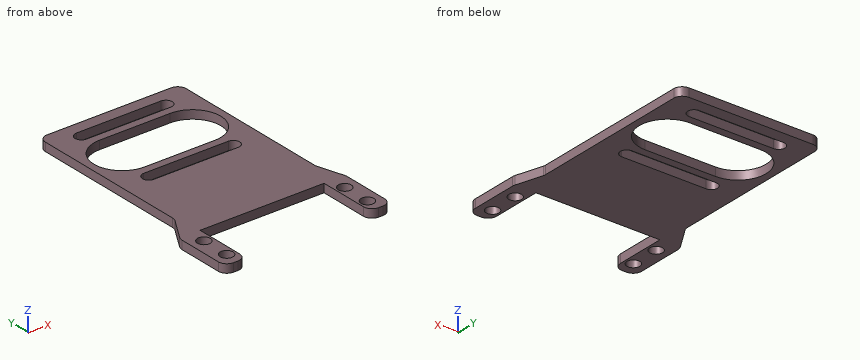
```python
from build123d import *

# Parameters (mm, degrees)
SKETCH1_R           = 2.3
BOSS_EXTRUDE1_DEPTH = 3
FILLET1_R           = 3


with BuildPart() as part:
    # Sketch1 → Boss-Extrude1 (new body)
    with BuildSketch(Plane.XY):
        Polygon((7.5, -20.05), (0, -20.05), (0, 0), (6, 10), (6, 70.5), (56, 70.5), (56, 10), (59, 0), (59, -20.05), (51.5, -20.05), (51.5, 0.5), (7.5, 0.5), align=None)
        with Locations((4.5, -15.05)):
            Circle(SKETCH1_R, mode=Mode.SUBTRACT)
        with Locations((4.5, -4.95)):
            Circle(SKETCH1_R, mode=Mode.SUBTRACT)
        with Locations((54.5, -15.05)):
            Circle(SKETCH1_R, mode=Mode.SUBTRACT)
        with Locations((54.5, -4.95)):
            Circle(SKETCH1_R, mode=Mode.SUBTRACT)
        with BuildLine():
            Line((18.5, 59), (43.5, 59))
            ThreePointArc((43.5, 59), (53.5, 49), (43.5, 39))
            Line((43.5, 39), (18.5, 39))
            ThreePointArc((18.5, 39), (8.5, 49), (18.5, 59))
        make_face(mode=Mode.SUBTRACT)
        with BuildLine():
            Line((16, 66.25), (46, 66.25))
            ThreePointArc((46, 66.25), (48.25, 64), (46, 61.75))
            Line((46, 61.75), (16, 61.75))
            ThreePointArc((16, 61.75), (13.75, 64), (16, 66.25))
        make_face(mode=Mode.SUBTRACT)
        with BuildLine():
            Line((16, 36.25), (46, 36.25))
            ThreePointArc((46, 36.25), (48.25, 34), (46, 31.75))
            Line((46, 31.75), (16, 31.75))
            ThreePointArc((16, 31.75), (13.75, 34), (16, 36.25))
        make_face(mode=Mode.SUBTRACT)
    extrude(amount=BOSS_EXTRUDE1_DEPTH)

    # Fillet1
    fillet1_edges = [part.edges().sort_by_distance(p)[0] for p in [
        (0, 0, 1.5),
        (6, 10, 1.5),
        (6, 70.5, 1.5),
        (56, 70.5, 1.5),
        (56, 10, 1.5),
        (59, 0, 1.5),
        (59, -20.05, 1.5),
        (51.5, -20.05, 1.5),
        (7.5, -20.05, 1.5),
        (0, -20.05, 1.5),
    ]]
    fillet(fillet1_edges, radius=FILLET1_R)


solid = part.part
```
CAD build for the part. Positions are in the model's coordinates, mm. Round coordinates to 2 decimals unless told otherwise and drop trailing zeros. Loops run counter-clockwise (first coordinate to the right, second up) from the corner with the lowest first, then second, coordinate; pieces in that order, holes last. Notation, with made-up numbers: M 58,-28.75 L 82,-28.75 A11 ccw 82,-24.75 Z; hole C 71,-18.75 d2. An arc over 180 degrees is marked long. Use a Markdown table: item, result. Add a question column.
(1) Cut at A-A (y = 64). Give the cut face in (x, z), and give its area (3 significant figures).
(2) Cut at B-B (x = 22.5). Give the cut face in (y, z).
(3) Cut at C-C (y = -4.95). Give the cut face in (x, z), and give its area (3 significant figures).
(4) Flat gauge pins, fed straight in: pin 1 (1.5 mm diameter, centred on x = 34, z = 1, fed in from -Y); pin 2 (3 mm diameter, centred on x = 4.5, y = -15.05, fed in from +Z); pin 3 (1.5 mm diameter, centred on y = 37.5, z = 2, fed in from -X). Where does each tip first touch, or does it go through?
(5) Drill centre lines: line 1 (Y direction, x = 36, z = 2.55); line 2 (Y direction, x = 4.5, z = 0.95); line 3 (X direction, y = -10, z = 1.15). Where is each one in solid material? Low to high.
(6) Cut at D-D (x = 10.5). Give the cut face in (y, z).
Geometry says:
| question | item | result |
|---|---|---|
| 1 | outline | M 6,0 L 13.75,0 L 13.75,3 L 6,3 Z; M 48.25,0 L 56,0 L 56,3 L 48.25,3 Z |
| 1 | area | 46.5 mm² |
| 2 | outline | M 0.5,0 L 31.75,0 L 31.75,3 L 0.5,3 Z; M 36.25,0 L 39,0 L 39,3 L 36.25,3 Z; M 59,0 L 61.75,0 L 61.75,3 L 59,3 Z; M 66.25,0 L 70.5,0 L 70.5,3 L 66.25,3 Z |
| 3 | outline | M 0,0 L 2.2,0 L 2.2,3 L 0,3 Z; M 6.8,0 L 7.5,0 L 7.5,3 L 6.8,3 Z; M 51.5,0 L 52.2,0 L 52.2,3 L 51.5,3 Z; M 56.8,0 L 59,0 L 59,3 L 56.8,3 Z |
| 3 | area | 17.4 mm² |
| 4 | pin 1 | stops at y = 0.5 |
| 4 | pin 2 | passes through |
| 4 | pin 3 | stops at x = 6 |
| 5 | line 1 | y = 0.5 to 31.75, 36.25 to 39, 59 to 61.75, 66.25 to 70.5 |
| 5 | line 2 | y = -20.05 to -17.35, -12.75 to -7.25, -2.65 to 7.5 |
| 5 | line 3 | x = 0 to 7.5, 51.5 to 59 |
| 6 | outline | M 0.5,0 L 43,0 L 43,3 L 0.5,3 Z; M 55,0 L 70.5,0 L 70.5,3 L 55,3 Z |
